For this review, take the finished solid that the model builds, in its own axes (mm). Give positions to 0.01 mm unless a question says otherwise; leave off trailing zeros. Order: outer loops, then holes, each group sorted by start corner. A loop starts at its lowest first (then second) coordinate and runs counter-clockwise, first axis right, second up. Notation, with made-up numbers: (-31.5, 68.25) - (-17.5, 68.25) arc R37 ccw to (-17.5, 106.25) - close; hole circle Ø8 at (51.5, 14.5). An arc over 180 degrees is marked (long way). Use a Markdown table: item, result. Add a question column.
1) Wall thickness on L1, parallel to X at y = 7, z = -2.75; L2, parallel to Y at x = 11, z = 2; L3, parallel to X at y = 6, z = -1.5: over which ranges is each line inside the solid? List them lowest first.
2) We need section D-D on z = -1.5. Write out the cut boundary in (x, y), then the cut area to 3 significant figures.
3) Clearance check with flat-ended pins moving along their axes: P1, Ø2, axis at y = 8, z = -1, coming from the +X side; P2, Ø3.5, axis at x = 11, y = 6, coming from the -Z side; P3, Ø1, axis at y = 3.5, z = 0.5, coming from the -X side. State where each tip first meets the part, or that it passes through.
4) We need section C-C on x = 12.75. Write out the cut boundary in (y, z), then the cut area to 3 significant figures.
5) We need section B-B on x = 11. Write out the cut boundary in (y, z), then the cut area to 3 significant figures.
6) We need section A-A on y = 6. Write out the cut boundary in (x, z), then the cut area to 3 significant figures.
Autodesk Inventor part; units mm, degrees
ref_plane "YZ Plane" through (0, 0, 0) normal (1, 0, 0) x (0, 1, 0)
ref_plane "XZ Plane" through (0, 0, 0) normal (0, 1, 0) x (-1, 0, 0)
ref_plane "XY Plane" through (0, 0, 0) normal (0, 0, 1) x (1, 0, 0)
sketch "Sketch1" plane through (0, 0, 0) normal (0, 0, 1) x (1, 0, 0)
  circle A0 centre (11, 6) radius 2
  circle A1 centre (11, 6) radius 1.5
  circle A2 centre (11, 6) radius 4
  line L0 (11, 10) -> (11, 1)
  point P0 (0, 0)
  point P1 (11, 2)
  dimension "d2" = 8
  dimension "d0" = 4
  dimension "d1" = 3
revolve "Revolution1" add sketch "Sketch1" angle 360 about axis through (11, 10, 0) along (0, -1, 0) picked at (12.8166, 5.8517) picked at (14.2832, 5.555) picked at (11.4875, 6.1113) contours A0 L0 A1 | A0 L0 A2 | A1 L0
extrude "Extrusion1" cut sketch "Sketch1" along normal mid plane 10 contours L0 A1 | A1 L0
extrude "Extrusion2" add sketch "Sketch1" along normal mid plane 7.5 contours A0 L0 A1 | L0 A1 A0
properties part number "bALL"
Checked values:
| question | item | result |
|---|---|---|
| 1 | L1 | 8.27 to 9.88, 12.12 to 13.73 |
| 1 | L2 | 2.54 to 4.5, 7.5 to 9.46 |
| 1 | L3 | 7.29 to 9.5, 12.5 to 14.71 |
| 2 | outline | circle Ø7.42 at (11, 6); hole circle Ø3 at (11, 6) |
| 2 | area | 36.1 mm² |
| 3 | P1 | x = 14.8 |
| 3 | P2 | z = -3.75 |
| 3 | P3 | x = 7.56 |
| 4 | outline | (5.03, -3.75) - (6.97, -3.75) - (6.97, -3.46) arc R3.6 ccw to (6.97, 3.46) - (6.97, 3.75) - (5.03, 3.75) - (5.03, 3.46) arc R3.6 ccw to (5.03, -3.46) - close |
| 4 | area | 41.4 mm² |
| 5 | outline | (4, -3.75) - (4.5, -3.75) - (4.5, 3.75) - (4, 3.75) - (4, 3.46) arc R4 ccw to (4, -3.46) - close; (7.5, -3.75) - (8, -3.75) - (8, -3.46) arc R4 ccw to (8, 3.46) - (8, 3.75) - (7.5, 3.75) - close |
| 5 | area | 27.2 mm² |
| 6 | outline | (9, -3.75) - (9.5, -3.75) - (9.5, 3.75) - (9, 3.75) - (9, 3.46) arc R4 ccw to (9, -3.46) - close; (12.5, -3.75) - (13, -3.75) - (13, -3.46) arc R4 ccw to (13, 3.46) - (13, 3.75) - (12.5, 3.75) - close |
| 6 | area | 27.2 mm² |
